Read the model definition and answer for the solid it produces. Units are mm, in the model's axes. A direction names the side the tool comes from. Coordinates: 2 decimals unless noted, no trailing zeros. Write each loop counter-clockwise with the first axis right and the second up, starting at its lowest first coordinate (ties: lowest second). Pieces come first, ordered by that corner, then holes.
1) The part is cut by section A-A (x = 25.4). Determine the outline of the cut face in (y, z) (1 decimal).
2) Find the intervals of material crossed by line 1 (Y direction, x = -44.5, z = -6.25); line 2 (Z direction, x = 80, y = -3); line 3 (X direction, y = -0.5, z = -1.5), in increasing order.
3) Determine the mould class of faces 3 (the face through (22.674, 6.261, 0.858)), 4 (the face through (25, 12.7, 0)), 5 (the face through (78.926, -18.961, 0.858)) for opening direction X: +X half, -X half, draft (parallel to the pull), parting line (faces both ways), or undercut.
4) Each of these flat-tipped pins is pushed along its axis until it touches: pin 1 Ø8 at (x, z) = (-31, -3) entering from +Y; pin 2 Ø8 at (x, y) = (-9.5, 6.5) entering from +Z; pin 3 Ø2 at (x, z) = (-26, 5) entering from -Y; pin 4 Ø6 at (y, z) = (-2, 7) entering from +X. Where does it stop, or does it pass through?
5) The part is cut by section D-D (y = 10). Determine the outline of the cut face in (x, z) (1 decimal), then the cut area to 3 significant figures.
6) The part is cut by section C-C (x = -50.8). Determine the outline of the cut face in (y, z) (1 decimal).
7) Which of the six approach directions +Z, -Z, +X, -X, +Y, -Y give full straight-line access (tool end or side, diameter ignored) to faces 1 (the face through (53.526, -18.961, 0.858)), 2 (the face through (-76, -25.4, 0))?
from build123d import *

# Parameters (mm, degrees)
F0_R     = 2.8575
F1_DEPTH = 12.7
F2_DEPTH = 25.4
F3_R     = 2.8575
F4_DEPTH = 12.7
F5_R     = 9.52499


# Not quite as in the source:
# - a fillet or chamfer is up to 0.001 mm smaller than in the source, because OpenCascade refuses the exact size
# - a feature names something its author has since deleted; it is built from what else it names


with BuildPart() as f1:
    # F0 (on Front) → F1 (new body)
    with BuildSketch(Plane.XZ):
        Polygon((-88.9, -9.525), (88.9, -9.525), (88.9, 9.525), (0, 9.525), (-88.9, 9.525), align=None)
        with Locations((-76.2, 0)):
            Circle(F0_R, mode=Mode.SUBTRACT)
        with Locations((-50.8, 0)):
            Circle(F0_R, mode=Mode.SUBTRACT)
        with Locations((-25.4, 0)):
            Circle(F0_R, mode=Mode.SUBTRACT)
        with BuildLine():
            ThreePointArc((2.8575, 0), (-2.0205576272, -2.0205576272), (0, 2.8575))
            ThreePointArc((0, 2.8575), (2.0205576272, 2.0205576272), (2.8575, 0))
        make_face(mode=Mode.SUBTRACT)
        with Locations((25.4, 0)):
            Circle(F0_R, mode=Mode.SUBTRACT)
        with Locations((50.8, 0)):
            Circle(F0_R, mode=Mode.SUBTRACT)
        with Locations((76.2, 0)):
            Circle(F0_R, mode=Mode.SUBTRACT)
    extrude(amount=F1_DEPTH)

    # F0 (on Front) → F2 (join)
    with BuildSketch(Plane.XZ):
        with BuildLine():
            ThreePointArc((2.8575, 0), (2.0205576272, 2.0205576272), (0, 2.8575))
            ThreePointArc((0, 2.8575), (-2.0205576272, -2.0205576272), (2.8575, 0))
        make_face()
        with Locations((-76.2, 0)):
            Circle(F0_R)
        with Locations((-50.8, 0)):
            Circle(F0_R)
        with Locations((-25.4, 0)):
            Circle(F0_R)
        with Locations((25.4, 0)):
            Circle(F0_R)
        with Locations((50.8, 0)):
            Circle(F0_R)
        with Locations((76.2, 0)):
            Circle(F0_R)
    extrude(amount=F2_DEPTH)

    # F3 (on face) → F4 (join)
    with BuildSketch(Plane(origin=(0, 0, 0), x_dir=(-1, 0, 0), z_dir=(0, 1, 0))):
        with Locations((-25.4, 0)):
            Circle(F3_R)
    extrude(amount=F4_DEPTH)

    # F5 (radius 9.525 in the source; OpenCascade refuses exactly that, so slightly less here)
    f5_edges = [f1.edges().sort_by_distance(p)[0] for p in [
        (88.9, -6.35, 9.525),
        (88.9, -6.35, -9.525),
        (-88.9, -6.35, -9.525),
        (-88.9, -6.35, 9.525),
    ]]
    fillet(f5_edges, radius=F5_R)


solid = f1.part
Reported:
1. outline: (-25.4, -2.9) - (-12.7, -2.9) - (-12.7, -9.5) - (0, -9.5) - (0, -2.9) - (12.7, -2.9) - (12.7, 2.9) - (0, 2.9) - (0, 9.5) - (-12.7, 9.5) - (-12.7, 2.9) - (-25.4, 2.9) - close
2. line 1: y = -12.7 to 0
2. line 2: z = -9.5 to 9.5
2. line 3: x = -88.78 to 88.78
3. face 3: parting line
3. face 4: draft
3. face 5: undercut
4. pin 1: stops at y = 0
4. pin 2: passes through
4. pin 3: stops at y = -12.7
4. pin 4: stops at x = 88.02
5. outline: circle Ø5.7 at (25.4, 0)
5. area: 25.7 mm2
6. outline: (-25.4, -2.9) - (-12.7, -2.9) - (-12.7, -9.5) - (0, -9.5) - (0, 9.5) - (-12.7, 9.5) - (-12.7, 2.9) - (-25.4, 2.9) - close
7. face 1: -Y
7. face 2: +Z, -Z, +X, -X, -Y
